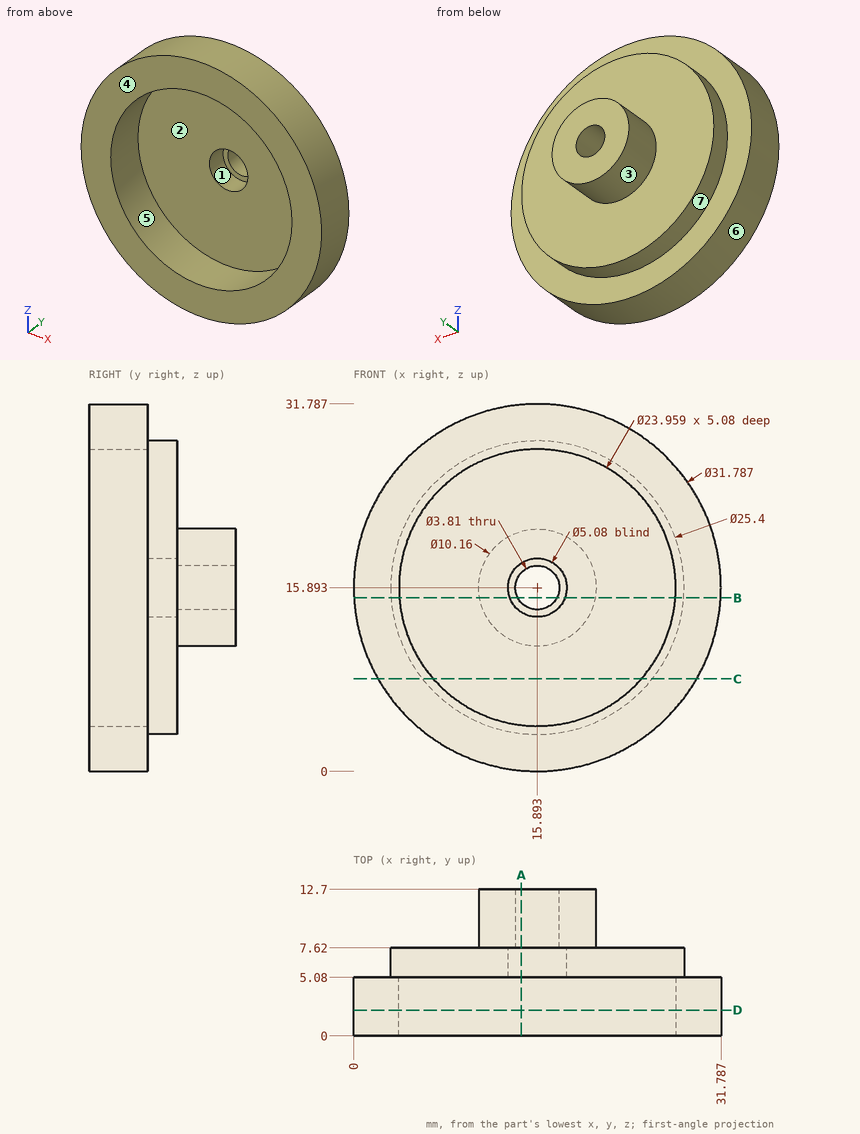
Drawing for the job (mm, zero at the part's lowest x, y, z). A direction names the side the tool comes from. Give positions to 0.01 mm unless a question says otherwise; leave off trailing zeros. Loops run counter-clockwise (first coordinate to the right, second up) from the corner with the lowest first, then second, coordinate; pieces in that order, holes last. Notation, with made-up numbers: M 17,48 L 67,48 A10 cw 67,53 Z; hole C 12,8.5 d11. An arc over 180 degrees is marked long. Use one line per item in the form item = value.
Item 1: Flat gauge pins, fed straight in: pin 1 (4 mm diameter, centred on x = 12.5, y = 6.5, fed in from -Z) (1 decimal); pin 2 (3 mm diameter, centred on y = 4.5, z = 20, fed in from -X) (1 decimal); pin 3 (6.5 mm diameter, centred on x = 15.89, z = 15.89, fed in from -Y); pin 4 (1.5 mm diameter, centred on x = 3, z = 8.5, fed in from -Y). Where does each tip first touch, or does it go through?
Determined:
pin_1 = 0.1
pin_2 = 0.2
pin_3 = 5.08
pin_4 = 0
Item 2: Two-plate mould, pull along X, no slides. Class the marked faces 1, 2, 3 and 4: pulls with the +X half, pulls with the -X half, needs draft (parallel to the pull), parting line crosses it, or undercut.
Determined:
face_1 = undercut
face_2 = undercut
face_3 = parting line crosses it
face_4 = needs draft
Item 3: Slice it at C-C (z = 8). List the corners of the cut face in (x, y) (1 decimal).
Determined:
outline = M 2.1,0 L 6.9,0 L 6.9,5.1 L 24.9,5.1 L 24.9,0 L 29.7,0 L 29.7,5.1 L 25.8,5.1 L 25.8,7.6 L 5.9,7.6 L 5.9,5.1 L 2.1,5.1 Z
Item 4: Which spindle directions (+Z, -Z, +X, -X, +Y, -Y) get a long thin tool onto all of the face, cutting with end or side? Do the marked faces 5, 6 and 7. Say none if no direction does.
Determined:
face_5 = -Y
face_6 = +Y, -Y
face_7 = +Y
Item 5: Slice it at D-D (y = 2.25). List the corners of the cut face in (x, z).
Determined:
outline = C 15.89,15.89 d31.79; hole C 15.89,15.89 d23.96
Item 6: Slice it at A-A (x = 14.5). List the corners of the cut face in (y, z) (1 decimal).
Determined:
outline = M 0,0.1 L 5.1,0.1 L 5.1,3.3 L 7.6,3.3 L 7.6,11 L 12.7,11 L 12.7,14.6 L 7.6,14.6 L 7.6,13.8 L 5.1,13.8 L 5.1,4 L 0,4 Z; M 0,27.8 L 5.1,27.8 L 5.1,18 L 7.6,18 L 7.6,17.2 L 12.7,17.2 L 12.7,20.8 L 7.6,20.8 L 7.6,28.5 L 5.1,28.5 L 5.1,31.7 L 0,31.7 Z
Item 7: Slice it at B-B (z = 15). List the corners of the cut face in (x, y) (1 decimal).
Determined:
outline = M 0,0 L 3.9,0 L 3.9,5.1 L 13.5,5.1 L 13.5,7.6 L 14.2,7.6 L 14.2,12.7 L 10.9,12.7 L 10.9,7.6 L 3.2,7.6 L 3.2,5.1 L 0,5.1 Z; M 17.6,7.6 L 18.3,7.6 L 18.3,5.1 L 27.8,5.1 L 27.8,0 L 31.8,0 L 31.8,5.1 L 28.6,5.1 L 28.6,7.6 L 20.9,7.6 L 20.9,12.7 L 17.6,12.7 Z
Item 8: Drill centre lines: probe 1 along Z at (x, y) = (15.5, 5) (1 decimal); probe 2 along Y at (x, z) = (13.5, 29); probe 3 along Y at (x, z) = (4.5, 16). Where is each one in solid material? Low to high. Write a range as from..to.
Determined:
probe_1 = 0..3.9, 27.9..31.8
probe_2 = 0..5.08
probe_3 = 5.08..7.62
